```python
from build123d import *

# Parameters (mm, degrees)
SALIENTE_EXTRUIR1_DEPTH    = 20
CROQUIS9_8_R               = 7.5
CORTAR_EXTRUIR1_DEPTH      = 20
CROQUIS9_10_R              = 7.5
CORTAR_EXTRUIR2_DEPTH      = 20
SALIENTE_EXTRUIR2_DEPTH    = 45
SALIENTE_EXTRUIR3_DEPTH    = 75
CORTAR_EXTRUIR4_DEPTH      = 61
CORTAR_EXTRUIR4_DEPTH_BACK = 52
CROQUIS12_R                = 6


with BuildPart() as part:
    # Croquis9 → Saliente-Extruir1 (new body)
    with BuildSketch(Plane.XY):
        with BuildLine():
            Line((-78, 14.696938457), (-6, 29.393876913))
            ThreePointArc((-6, 29.393876913), (0, 30), (6, 29.393876913))
            Line((6, 29.393876913), (78, 14.696938457))
            ThreePointArc((78, 14.696938457), (90, 0), (78, -14.696938457))
            Line((78, -14.696938457), (6, -29.393876913))
            ThreePointArc((6, -29.393876913), (0, -30), (-6, -29.393876913))
            Line((-6, -29.393876913), (-78, -14.696938457))
            ThreePointArc((-78, -14.696938457), (-90, 0), (-78, 14.696938457))
        make_face()
    extrude(amount=SALIENTE_EXTRUIR1_DEPTH)

    # Croquis9_8 → Cortar-Extruir1 (cut)
    with BuildSketch(Plane.XY):
        with Locations((-75, 0)):
            Circle(CROQUIS9_8_R)
    extrude(amount=CORTAR_EXTRUIR1_DEPTH, mode=Mode.SUBTRACT)

    # Croquis9_10 → Cortar-Extruir2 (cut)
    with BuildSketch(Plane.XY):
        with Locations((75, 0)):
            Circle(CROQUIS9_10_R)
    extrude(amount=CORTAR_EXTRUIR2_DEPTH, mode=Mode.SUBTRACT)

    # Croquis10 → Saliente-Extruir2 (add)
    with BuildSketch(Plane.XY):
        with BuildLine():
            Line((-29.047375097, 7.5), (29.047375097, 7.5))
            ThreePointArc((29.047375097, 7.5), (0, 30), (-29.047375097, 7.5))
        make_face()
        with BuildLine():
            Line((-29.047375097, -7.5), (29.047375097, -7.5))
            ThreePointArc((29.047375097, -7.5), (0, -30), (-29.047375097, -7.5))
        make_face()
    extrude(amount=SALIENTE_EXTRUIR2_DEPTH)

    # Croquis11 → Saliente-Extruir3 (add)
    with BuildSketch(Plane.XY):
        with BuildLine():
            Line((-24.366985862, 17.5), (24.366985862, 17.5))
            ThreePointArc((24.366985862, 17.5), (27.171188586, 12.717173855), (29.047375097, 7.5))
            Line((29.047375097, 7.5), (-29.047375097, 7.5))
            ThreePointArc((-29.047375097, 7.5), (-27.171188586, 12.717173855), (-24.366985862, 17.5))
        make_face()
        with BuildLine():
            Line((-24.366985862, -17.5), (24.366985862, -17.5))
            ThreePointArc((24.366985862, -17.5), (27.171188586, -12.717173855), (29.047375097, -7.5))
            Line((29.047375097, -7.5), (-29.047375097, -7.5))
            ThreePointArc((-29.047375097, -7.5), (-27.171188586, -12.717173855), (-24.366985862, -17.5))
        make_face()
    extrude(amount=SALIENTE_EXTRUIR3_DEPTH)

    # Croquis12 → Cortar-Extruir4 (cut, two sides: drawn at the far end of the back side and taken through both)
    with BuildSketch(Plane(origin=(0, 0, 0), x_dir=(1, 0, 0), z_dir=(0, 1, 0)).offset(-CORTAR_EXTRUIR4_DEPTH_BACK)):
        with Locations(Location((0, -60, 0), (0, 0, 90))):
            Circle(CROQUIS12_R)
    extrude(amount=CORTAR_EXTRUIR4_DEPTH + CORTAR_EXTRUIR4_DEPTH_BACK, mode=Mode.SUBTRACT)


solid = part.part
```
Source: CAD feature listing. Evaluate the final solid. Frame: model axes, mm. A direction names the side the tool comes from. Give positions to 0.01 mm unless a question says otherwise; leave off trailing zeros. Write each loop counter-clockwise with the first axis right and the second up, starting at its lowest first coordinate (ties: lowest second). Pieces come first, ordered by that corner, then holes.
1. Section query C-C (y = 0). Return the cut outline in (x, z), then the cut area to 3 significant figures.
2. Access query for faces 1 (the face through (0, 22, 45)), 2 (the face through (-6, -17.5, 56)), 3 (the face through (0, 7.5, 47)). Directions: +Z, -Z, +X, -X, +Y, -Y. A direction counts if a zero-diameter tool reaches every point of the face in a straight line with its end or side. Return the directions, or none.
3. Section query A-A (z = 12.5). Return the cut outline in (x, y), then the cut area to 3 significant figures.
4. Material intervals for line 1 along X through (y, z) = (-2.5, 11); line 2 along Z through (x, y) = (50, -14); line 3 along Z through (x, y) = (20, -20.5), sorted ascending.
5. Pull-direction query (Y, two-part tool) for faces 4 (the face through (-0.554, 29.995, 36.975)), 5 (the face through (0, -7.5, 47)), 6 (the face through (0, -22, 45)); classes: +Y half, -Y half, draft (parallel to the pull), parting line (faces both ways), or undercut.
6. First-contact query: pin 1 (13.5 mm diameter, centred on x = -11, y = -24.5, fed in from +Z); pin 2 (5 mm diameter, centred on y = -13, z = 20.5, fed in from -X); pin 3 (9 mm diameter, centred on x = -8.5, z = 65, fed in from +Y); pin 4 (13.5 mm diameter, centred on x = -75, y = 0, fed in from -Z). Flat tips, straight axial feed; report the tip coordinate or a pass-through.
7. Section query B-B (x = 75). Return the cut outline in (y, z).
8. Section query D-D (z = 47.5). Return the cut outline in (x, y), then the cut area to 3 significant figures.
Output values:
1. outline: (-90, 0) - (-82.5, 0) - (-82.5, 20) - (-90, 20) - close; (-67.5, 0) - (67.5, 0) - (67.5, 20) - (-67.5, 20) - close; (82.5, 0) - (90, 0) - (90, 20) - (82.5, 20) - close
1. area: 3,000 mm2
2. face 1: +Z, +X, -X, +Y
2. face 2: +Z, +X, -X, -Y
2. face 3: +Z, +X, -X
3. outline: (-78, -14.7) - (-6, -29.39) arc R30 ccw to (6, -29.39) - (78, -14.7) arc R15 ccw to (78, 14.7) - (6, 29.39) arc R30 ccw to (-6, 29.39) - (-78, 14.7) arc R15 ccw to start; hole circle Ø15 at (-75, 0); hole circle Ø15 at (75, 0)
3. area: 7,240 mm2
4. line 1: x = -89.79 to -82.07, -67.93 to 67.93, 82.07 to 89.79
4. line 2: z = 0 to 20
4. line 3: z = 0 to 45
5. face 4: +Y half
5. face 5: undercut
5. face 6: draft
6. pin 1: stops at z = 45
6. pin 2: stops at x = -85.66
6. pin 3: stops at y = 17.5
6. pin 4: passes through
7. outline: (-15.31, 0) - (-7.5, 0) - (-7.5, 20) - (-15.31, 20) - close; (7.5, 0) - (15.31, 0) - (15.31, 20) - (7.5, 20) - close
8. outline: (-29.05, -7.5) arc R30 ccw to (-24.37, -17.5) - (24.37, -17.5) arc R30 ccw to (29.05, -7.5) - close; (-29.05, 7.5) - (29.05, 7.5) arc R30 ccw to (24.37, 17.5) - (-24.37, 17.5) arc R30 ccw to start
8. area: 1,080 mm2
